Can you work these out from the model? Positions are in its coordinate system, mm. A direction names the side the tool comes from. Give positions to 0.01 mm unless a question says otherwise; leave off trailing zeros. Loops run counter-clockwise (first coordinate to the right, second up) from the corner with the lowest first, then second, coordinate; pieces in that order, holes last.
from build123d import *


with BuildPart() as part:
    # Esquisse2 → Base-Révolution (revolve)
    with BuildSketch(Plane(origin=(0, 0, 0), x_dir=(1, 0, 0), z_dir=(0, 1, 0)), mode=Mode.PRIVATE) as base_r_volution_sk:
        Polygon((-16.680780303, -30.626231876), (-16.680780303, -10.599160722), (-16.480780303, -10.599160722), (-16.480780303, -9.599160722), (-16.680780303, -9.599160722), (-16.680780303, -9.099160722), (-15.680780303, -8.099160722), (-12.680780303, -8.099160722), (-12.680780303, -43.599160722), (-18.680780303, -43.599160722), (-19.680780303, -42.599160722), (-19.680780303, -40.599160722), (-16.680780303, -40.599160722), align=None)
    revolve(base_r_volution_sk.sketch.rotate(Axis((-12.680780303, 0, 67.53791491), (0, 0, -1)), 180), axis=Axis((-12.680780303, 0, 67.53791491), (0, 0, -1)))


solid = part.part
(1) Suppose I cut it at B-B on z = 37. List the corners of the cut face in (x, y) for me.
Returned:
outline: circle Ø8 at (-12.68, 0)
(2) Thinking about a two-plate mould opening in Z: for faces 1 (the flat face through (-13, 0, 43.599)), 2 (the cylindrical face through (-16.477, -0.167, 10.092)), 3 (the cylindrical face through (-8.865, -1.201, 25.809)), which applies, pulls with the +Z half, pulls with the -Z half, needs draft (parallel to the pull), parting line crosses it, or undercut?
Returned:
face 1: pulls with the +Z half
face 2: undercut
face 3: needs draft
(3) Suppose I cut it at A-A on y = 0. List the corners of the cut face in (x, z) for me.
Returned:
outline: (-19.68, 40.6) - (-16.68, 40.6) - (-16.68, 10.6) - (-16.48, 10.6) - (-16.48, 9.6) - (-16.68, 9.6) - (-16.68, 9.1) - (-15.68, 8.1) - (-9.68, 8.1) - (-8.68, 9.1) - (-8.68, 9.6) - (-8.88, 9.6) - (-8.88, 10.6) - (-8.68, 10.6) - (-8.68, 40.6) - (-5.68, 40.6) - (-5.68, 42.6) - (-6.68, 43.6) - (-18.68, 43.6) - (-19.68, 42.6) - close
(4) Will these pins go through, and if not, where does the flat tip stop? P1, Ø5, axis at x = -15.5, z = 33.5, coming from the -Y side; P2, Ø8, axis at x = -16.5, z = 19, coming from the +Y side; P3, Ø8, axis at y = 3, z = 37.5, coming from the +X side; P4, Ø4, axis at x = -16, y = -2, coming from the -Z side.
Returned:
P1: stops at y = -3.99
P2: stops at y = 4
P3: stops at x = -5.7
P4: stops at z = 8.1
(5) Please list where these lines run through material, in increasing order: probe 1 along Z at (x, y) = (-8, -2.25); probe 2 along X at (y, z) = (1.25, 17); probe 3 along X at (y, z) = (-3, 21.5).
Returned:
probe 1: z = 40.6 to 43.6
probe 2: x = -16.48 to -8.88
probe 3: x = -15.33 to -10.04
(6) Which directions (+Z, -Z, +X, -X, +Y, -Y) give clear straight access to the entire face, cutting with the end or side of a thin tool? Please do faces 4 (the flat face through (-13, 0, 8.099)), 5 (the cylindrical face through (-8.865, -1.201, 9.346)).
Returned:
face 4: -Z, +X, -X, +Y, -Y
face 5: -Z
